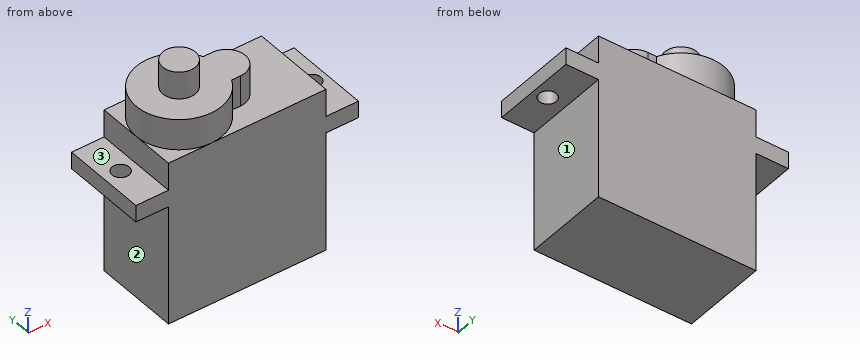
from build123d import *

# Parameters (mm, degrees)
SKETCH_1_W          = 23
SKETCH_1_H          = 12.5
EXTRUDE_1_DEPTH     = 24
SKETCH_2_W          = 32.5
SKETCH_2_H          = 12.5
EXTRUDE_2_DEPTH     = 2.46
EXTRUDE_3_DEPTH     = 4.5
SKETCH_4_R          = 2.381232182
EXTRUDE_4_DEPTH     = 4
SKETCH_6_R          = 1.25
CUT_EXTRUDE_1_DEPTH = 37.396622096


with BuildPart() as part:
    # 草图1 → 凸台-拉伸1 (new body)
    with BuildSketch(Plane.XY):
        with Locations((11.5, -6.25)):
            Rectangle(SKETCH_1_W, SKETCH_1_H)
    extrude(amount=EXTRUDE_1_DEPTH)

    # 草图2 → 凸台-拉伸2 (add)
    with BuildSketch(Plane.XY.offset(17.5)):
        with Locations((11.5, -6.25)):
            Rectangle(SKETCH_2_W, SKETCH_2_H)
    extrude(amount=EXTRUDE_2_DEPTH)

    # 草图3 → 凸台-拉伸3 (add)
    with BuildSketch(Plane.XY.offset(24)):
        with BuildLine():
            Line((13.167793033, -3.5), (11.86248608, -3.5))
            ThreePointArc((11.86248608, -3.5), (0, -6.25), (11.86248608, -9))
            Line((11.86248608, -9), (13.167793033, -9))
            ThreePointArc((13.167793033, -9), (15.917793033, -6.25), (13.167793033, -3.5))
        make_face()
    extrude(amount=EXTRUDE_3_DEPTH)

    # 草图4 → 凸台-拉伸4 (add)
    with BuildSketch(Plane.XY.offset(28.5)):
        with Locations((6.25, -6.25)):
            Circle(SKETCH_4_R)
    extrude(amount=EXTRUDE_4_DEPTH)

    # 草图6 → 切除-拉伸1 (cut, through all)
    with BuildSketch(Plane.XY.offset(19.96)):
        with Locations((-2.286532447, -6.25)):
            Circle(SKETCH_6_R)
        with Locations((25.713467553, -6.25)):
            Circle(SKETCH_6_R)
    extrude(amount=-CUT_EXTRUDE_1_DEPTH, mode=Mode.SUBTRACT)


solid = part.part
Can you work these out from the model? Positions are in its coordinate system, mm. Face numbers are marked on the shaded views. A direction names the side the tool comes from. Give positions to 0.01 mm unless a question says otherwise; leave off trailing zeros. Loops run counter-clockwise (first coordinate to the right, second up) from the corner with the lowest first, then second, coordinate; pieces in that order, holes last. Notation, with made-up numbers: (52.25, -35.75) -> (103.25, -35.75) arc R19 ccw to (103.25, -0.75) -> close; hole circle Ø2 at (49.25, 79.25). An arc over 180 degrees is marked (long way). Use one line per item in the form item = value.
1) I need wall thicknesses on line 1 along Z through (x, y) = (25.5, -9); line 2 along Z through (x, y) = (4.5, -9.25); line 3 along X through (y, z) = (-11.25, 23). Which ranges of each line are inside material? Lowest first, please.
Answers:
line_1 = 17.5 to 19.96
line_2 = 0 to 28.5
line_3 = 0 to 23
2) If we section it at A-A (x = 8): Please give me the cut outline in (y, z).
Answers:
outline = (-12.5, 0) -> (0, 0) -> (0, 24) -> (-0.25, 24) -> (-0.25, 28.5) -> (-4.64, 28.5) -> (-4.64, 32.5) -> (-7.86, 32.5) -> (-7.86, 28.5) -> (-12.25, 28.5) -> (-12.25, 24) -> (-12.5, 24) -> close
3) If we section it at C-C (z = 25.5): Please give me the cut outline in (x, y), plus the area to 3 significant figures.
Answers:
outline = (11.86, -9) -> (13.17, -9) arc R2.75 ccw to (13.17, -3.5) -> (11.86, -3.5) arc R6.25 ccw (long way) to start
area = 139 mm²
4) Will these pins go through, and if not, where does the flat tip stop? pin 1 (3 mm diameter, centred on x = 3.5, y = -2, fed in from +Z); pin 2 (4 mm diameter, centred on x = 8.5, y = -8.5, fed in from +Z); pin 3 (4 mm diameter, centred on x = -2.5, y = -9, fed in from +Z); pin 4 (1 mm diameter, centred on x = 12.5, z = 26, fed in from +Y).
Answers:
pin_1 = 28.5
pin_2 = 32.5
pin_3 = 19.96
pin_4 = -3.5
5) If we section it at B-B (z = 11): Please give me the cut outline in (x, y), plus the area to 4 significant figures.
Answers:
outline = (0, -12.5) -> (23, -12.5) -> (23, 0) -> (0, 0) -> close
area = 287.5 mm²
6) For the marked faces 1, 2 and 3, which set-ups out of +Z, -Z, +X, -X, +Y, -Y let a thin tool reach every point of the face, with its end or its side?
Answers:
face_1 = -Z, +X, +Y, -Y
face_2 = -Z, -X, +Y, -Y
face_3 = +Z, -X, +Y, -Y
